from build123d import *

# Parameters (mm, degrees)
F0_R     = 2.5
F0_R_2   = 7
F0_R_3   = 15
F0_R_4   = 10
F1_DEPTH = 6
F2_SIZE  = 3.1


with BuildPart() as f1:
    # F0 (on Front) → F1 (new body)
    with BuildSketch(Plane.XZ):
        with BuildLine():
            Line((37.689998, 25), (0, 25))
            ThreePointArc((0, 25), (-24.573155, -4.600004), (9.042928, -23.307197))
            Line((9.042928, -23.307197), (18.961279, -19.45899))
            ThreePointArc((18.961279, -19.45899), (26.3962, -17.817954), (33.98027, -18.49096))
            Line((33.98027, -18.49096), (67.13149, -26.652109))
            ThreePointArc((67.13149, -26.652109), (80.508551, -20.793993), (78.322499, -6.355001))
            Line((78.322499, -6.355001), (51.56083, 19.408331))
            ThreePointArc((51.56083, 19.408331), (45.167744, 23.549483), (37.689998, 25))
        make_face()
        with Locations((27.055728, -9.404564)):
            Circle(F0_R, mode=Mode.SUBTRACT)
        with Locations((44.944272, -15.216904)):
            Circle(F0_R, mode=Mode.SUBTRACT)
        with Locations((70, -15)):
            Circle(F0_R_2, mode=Mode.SUBTRACT)
        Circle(F0_R_3, mode=Mode.SUBTRACT)
        with Locations((27.055728, 9.404564)):
            Circle(F0_R, mode=Mode.SUBTRACT)
        with Locations((40, 0)):
            Circle(F0_R_4, mode=Mode.SUBTRACT)
        with Locations((56, 0)):
            Circle(F0_R, mode=Mode.SUBTRACT)
        with Locations((44.944272, 15.216904)):
            Circle(F0_R, mode=Mode.SUBTRACT)
    extrude(amount=F1_DEPTH)

    # F2
    f2_edges = [f1.edges().sort_by_distance(p)[0] for p in [
        (24.555728, -6, -9.404564),
        (24.555728, -6, 9.404564),
        (42.444272, -6, 15.216904),
        (53.5, -6, 0),
        (42.444272, -6, -15.216904),
    ]]
    chamfer(f2_edges, length=F2_SIZE)


solid = f1.part
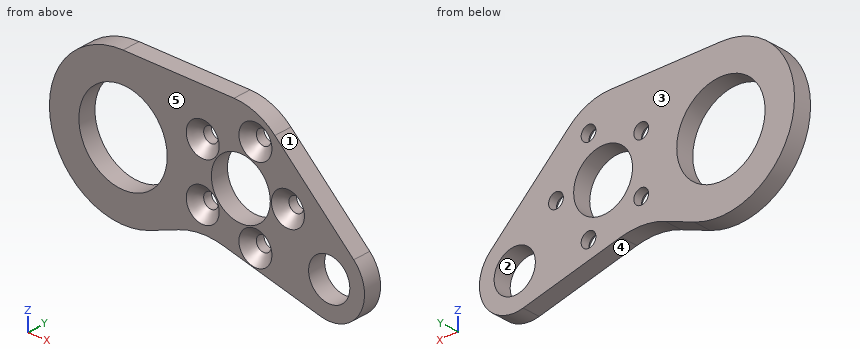
Could you check a few things on this model? Use its own coordinates, in mm. Face numbers are marked on the shaded views. A direction names the side the tool comes from. Give positions to 0.01 mm unless a question says otherwise; leave off trailing zeros. Write each loop counter-clockwise with the first axis right and the second up, starting at its lowest first coordinate (ties: lowest second). Pieces come first, ordered by that corner, then holes. Notation, with made-up numbers: (-13.5, 87) -> (14.5, 87) arc R29 cw to (14.5, 123) -> close; hole circle Ø4 at (75.25, -17.5). An arc over 180 degrees is marked (long way). Write each question's results on one line, items separated by ' | '. Start each with the question number.
Q1. Which directions (+Z, -Z, +X, -X, +Y, -Y) give clear straight access to the entire face, cutting with the end or side of a thin tool? Please do the marked faces 4 and 5.
Q2. I'm going to push flat-ended pins straight in: pin 1 Ø3 at (y, z) = (-4, -7) entering from +X; pin 2 Ø1 at (y, z) = (-3, -0.5) entering from +X; pin 3 Ø6.5 at (x, z) = (27.06, 9.4) entering from -Y. Where does each tip first touch, or does it pass through?
Q3. Suppose I cut it at D-D, the plane x = 56. List the corners of the cut face in (y, z) for me.
Q4. Suppose I cut it at C-C, the plane y = -1.45. State how many separate pieces and enclosed holes the cut face has, and give its area (3 significant figures).
Q5. Suppose I cut it at A-A, the plane x = 70.5. List the corners of the cut face in (y, z) for me.
Q6. Suppose I cut it at B-B, the plane z = 0. List the corners of the cut face in (x, y) for me.
Q7. We'd pull the mould along X, two halves only. Please class the marked faces 1, 2 and 3: +X half, -X half, draft (parallel to the pull), parting line (faces both ways), or undercut.
Q8. I need wall thicknesses on probe 1 along X at (y, z) = (-4.35, -12); probe 2 along X at (y, z) = (-1.85, -3.5); probe 3 along X at (y, z) = (-2.45, 4.5). Which ranges of each line are inside material? Lowest first, please.
Outcome:
1) face 4: -Z, +Y, -Y | face 5: +Z, -Z, +X, -X, -Y
2) pin 1: x = 80.09 | pin 2: x = 72.76 | pin 3: y = -3.66
3) outline: (-6, -23.91) -> (0, -23.91) -> (0, -2.5) -> (-2.9, -2.5) -> (-6, -5.6) -> close; (-6, 5.6) -> (-2.9, 2.5) -> (0, 2.5) -> (0, 15.13) -> (-6, 15.13) -> close
4) separate pieces: 1 | enclosed holes: 8 | area: 2,940 mm2
5) outline: (-6, -26.99) -> (0, -26.99) -> (0, -21.98) -> (-6, -21.98) -> close; (-6, -8.02) -> (0, -8.02) -> (0, 1.18) -> (-6, 1.18) -> close
6) outline: (-25, -6) -> (-15, -6) -> (-15, 0) -> (-25, 0) -> close; (15, -6) -> (30, -6) -> (30, 0) -> (15, 0) -> close; (50, -6) -> (50.4, -6) -> (53.5, -2.9) -> (53.5, 0) -> (50, 0) -> close; (58.5, -2.9) -> (61.6, -6) -> (71.72, -6) -> (71.72, 0) -> (58.5, 0) -> close
7) face 1: +X half | face 2: undercut | face 3: draft
8) probe 1: -21.93 to -9, 9 to 24.08, 30.03 to 42.65, 47.24 to 63.68, 76.32 to 81.62 | probe 2: -24.75 to -14.59, 14.59 to 30.63, 49.37 to 75.36 | probe 3: -24.59 to -14.31, 14.31 to 31.07, 48.93 to 67.05
